from build123d import *

# Parameters (mm, degrees)
SKETCH_1_W                  = 65
SKETCH_1_H                  = 40
EXTRUDE_1_DEPTH             = 6
SKETCH_2_W                  = 48
SKETCH_2_H                  = 1.5
CUT_EXTRUDE_1_DEPTH         = 77.557168182
HOLE_WIZARD_3_5_3_5_1_D     = 3.5
HOLE_WIZARD_3_5_3_5_1_DEPTH = 10
HOLE_WIZARD_3_5_3_5_1_TIP   = 1.051506083
HOLE_WIZARD_M3_1_D          = 2.5
SKETCH_7_W                  = 30
SKETCH_7_H                  = 24
CUT_EXTRUDE_2_DEPTH         = 10
SKETCH_9_W                  = 15
SKETCH_9_H                  = 14
CUT_EXTRUDE_3_DEPTH         = 77.557168182


with BuildPart() as part:
    # 草图1 → 凸台-拉伸1 (new body)
    with BuildSketch(Plane.XY):
        with Locations((32.5, 20)):
            Rectangle(SKETCH_1_W, SKETCH_1_H)
    extrude(amount=EXTRUDE_1_DEPTH)

    # 草图2 → 切除-拉伸1 (cut, through all)
    with BuildSketch(Plane(origin=(0, 40, 0), x_dir=(1, 0, 0), z_dir=(0, 1, 0))):
        with Locations((24, -0.75)):
            Rectangle(SKETCH_2_W, SKETCH_2_H)
    extrude(amount=-CUT_EXTRUDE_1_DEPTH, mode=Mode.SUBTRACT)

    # Ø3.5 (3.5) 直径孔1
    with Locations(Plane.XY.offset(6)):
        with Locations((25, 31.5), (5, 31.5)):
            Hole(HOLE_WIZARD_3_5_3_5_1_D / 2, depth=HOLE_WIZARD_3_5_3_5_1_DEPTH)
            with Locations((0, 0, -(HOLE_WIZARD_3_5_3_5_1_DEPTH + HOLE_WIZARD_3_5_3_5_1_TIP / 2))):  # 118° drill point
                Cone(0, HOLE_WIZARD_3_5_3_5_1_D / 2, HOLE_WIZARD_3_5_3_5_1_TIP, mode=Mode.SUBTRACT)

    # M3 螺纹孔1 (through all)
    with Locations(Plane.XY.offset(6)):
        with Locations((50.2, 8), (50.2, 24)):
            Hole(HOLE_WIZARD_M3_1_D / 2)

    # 草图7 → 切除-拉伸2 (cut)
    with BuildSketch(Plane.XY.offset(6)):
        with Locations((15, 12)):
            Rectangle(SKETCH_7_W, SKETCH_7_H)
    extrude(amount=-CUT_EXTRUDE_2_DEPTH, mode=Mode.SUBTRACT)

    # 草图9 → 切除-拉伸3 (cut, through all)
    with BuildSketch(Plane.XY.offset(6)):
        with Locations((57.5, 33)):
            Rectangle(SKETCH_9_W, SKETCH_9_H)
    extrude(amount=-CUT_EXTRUDE_3_DEPTH, mode=Mode.SUBTRACT)


solid = part.part
CAD build for the part. Positions are in the model's coordinates, mm. A direction names the side the tool comes from. Round coordinates to 2 decimals unless told otherwise and drop trailing zeros. Write each loop counter-clockwise with the first axis right and the second up, starting at its lowest first coordinate (ties: lowest second). Pieces come first, ordered by that corner, then holes.
(1) Drop flat-ended pins along their axis: P1, Ø2, axis at x = 50.2, y = 24, coming from the +Z side; P2, Ø2, axis at x = 12, z = 3.5, coming from the -Y side; P3, Ø1.3, axis at y = 15.5, z = 3, coming from the -X side; P4, Ø3, axis at x = 55, z = 3.5, coming from the +Y side. Give the stop position or say it passes through.
(2) 3-axis set-ups, long thin cutter, end or side, ignore diameter. For faces 4 (the face through (30, 12, 4)), 5 (the face through (48, 20, 1)), 6 (the face through (50, 33, 3)), 7 (the face through (26.75, 31.58, 3.72)), 8 (the face through (39, 20, 6)): which of +Z, -Z, +X, -X, +Y, -Y reach the whole face in a straight line?
(3) Slice it at B-B, the plane x = 5. Write the cut outline in (y, z), and give its area (4 significant figures).
(4) Slice it at C-C, the plane y = 3.5. Write the cut outline in (x, z), and give its area (3 significant figures).
(5) Probe line 1 along Y through (x, z) = (50.2, 2.9); line 2 along Y through (x, z) = (5, 4.45); line 3 along Z through (x, y) = (6.5, 27). List the from-to ranges inside material, lowest first.
(6) Slice it at A-A, the plane z = 3.85. Write the cut outline in (x, y).
(7) Mould opens along Y. For faces 1 (the face through (65, 13, 3)), 2 (the face through (57, 26, 3)), 3 (the face through (6.29, 32.68, 3.72)) say: pulls with the +Y half, pulls with the -Y half, needs draft (parallel to the pull), parting line crosses it, or undercut.
(8) Slice it at D-D, the plane x = 24.5. Write the cut outline in (y, z), and give its area (3 significant figures).
From the geometry:
1. P1: passes through
1. P2: stops at y = 24
1. P3: stops at x = 30
1. P4: stops at y = 26
2. face 4: +Z, -Z, -X, -Y
2. face 5: -Z, -X, +Y, -Y
2. face 6: +Z, -Z, +X, +Y
2. face 7: +Z, -Z
2. face 8: +Z, +X, -X, +Y, -Y
3. outline: (24, 1.5) - (29.75, 1.5) - (29.75, 6) - (24, 6) - close; (33.25, 1.5) - (40, 1.5) - (40, 6) - (33.25, 6) - close
3. area: 56.25 mm2
4. outline: (30, 1.5) - (48, 1.5) - (48, 0) - (65, 0) - (65, 6) - (30, 6) - close
4. area: 183 mm2
5. line 1: y = 0 to 6.75, 9.25 to 22.75, 25.25 to 26
5. line 2: y = 24 to 29.75, 33.25 to 40
5. line 3: z = 1.5 to 6
6. outline: (0, 24) - (30, 24) - (30, 0) - (65, 0) - (65, 26) - (50, 26) - (50, 40) - (0, 40) - close; hole circle Ø3.5 at (5, 31.5); hole circle Ø3.5 at (25, 31.5); hole circle Ø2.5 at (50.2, 8); hole circle Ø2.5 at (50.2, 24)
7. face 1: needs draft
7. face 2: pulls with the +Y half
7. face 3: undercut
8. outline: (24, 1.5) - (29.82, 1.5) - (29.82, 6) - (24, 6) - close; (33.18, 1.5) - (40, 1.5) - (40, 6) - (33.18, 6) - close
8. area: 56.9 mm2
